```python
from build123d import *

# Parameters (mm, degrees)
SKETCH1_W           = 55
SKETCH1_H           = 13
BOSS_EXTRUDE1_DEPTH = 5
SKETCH2_R           = 4
BOSS_EXTRUDE2_DEPTH = 13
CUT_EXTRUDE1_REACH  = 63.016
SKETCH3_R           = 2.3


with BuildPart() as part:
    # Sketch1 → Boss-Extrude1 (new body)
    with BuildSketch(Plane(origin=(0, 0, 0), x_dir=(1, 0, 0), z_dir=(0, 1, 0))):
        with Locations((27.5, 6.5)):
            Rectangle(SKETCH1_W, SKETCH1_H)
    extrude(amount=BOSS_EXTRUDE1_DEPTH)

    # Sketch2 → Boss-Extrude2 (add)
    with BuildSketch(Plane.XY):
        with BuildLine():
            Line((13.5, 14), (13.5, 0))
            Line((13.5, 0), (41.5, 0))
            Line((41.5, 0), (41.5, 14))
            ThreePointArc((41.5, 14), (27.5, 28), (13.5, 14))
        make_face()
        with Locations((27.5, 14)):
            Circle(SKETCH2_R, mode=Mode.SUBTRACT)
    extrude(amount=-BOSS_EXTRUDE2_DEPTH)

    # Sketch3 → Cut-Extrude1 (cut, up to next)
    with BuildSketch(Plane(origin=(0, 5, 0), x_dir=(1, 0, 0), z_dir=(0, 1, 0)), mode=Mode.PRIVATE) as cut_extrude1_sk1:
        with Locations(Location((48.5, 6.5, 0), (0, 0, 270))):
            Circle(SKETCH3_R)
    cut_extrude1_tool1 = extrude(cut_extrude1_sk1.sketch, amount=-CUT_EXTRUDE1_REACH, mode=Mode.PRIVATE) & part.part
    # Sketch3 → Cut-Extrude1 (cut, up to next)
    with BuildSketch(Plane(origin=(0, 5, 0), x_dir=(1, 0, 0), z_dir=(0, 1, 0)), mode=Mode.PRIVATE) as cut_extrude1_sk2:
        with Locations(Location((6.5, 6.5, 0), (0, 0, 270))):
            Circle(SKETCH3_R)
    cut_extrude1_tool2 = extrude(cut_extrude1_sk2.sketch, amount=-CUT_EXTRUDE1_REACH, mode=Mode.PRIVATE) & part.part
    add(cut_extrude1_tool1.solids().sort_by_distance((48.5, 5, -6.5))[0], mode=Mode.SUBTRACT)
    add(cut_extrude1_tool2.solids().sort_by_distance((6.5, 5, -6.5))[0], mode=Mode.SUBTRACT)


solid = part.part
```
Read the model definition and answer for the solid it produces. Units are mm, in the model's axes. A direction names the side the tool comes from. Give positions to 0.01 mm unless a question says otherwise; leave off trailing zeros. Write each loop counter-clockwise with the first axis right and the second up, starting at its lowest first coordinate (ties: lowest second). Pieces come first, ordered by that corner, then holes. Notation, with made-up numbers: (72.25, 84) - (126.25, 84) arc R18 cw to (126.25, 91) - close; hole circle Ø8 at (21.5, 26). An arc over 180 degrees is marked (long way). Write item = value, one per line. Start each with the question number.
Item 1: Find section C-C (y = 11.25). Give the vertices of the cut face in (x, z).
Item 2: Each of these flat-tipped pins is pushed along its axis until it touches: P1, Ø4, axis at x = 46.5, z = -4.5, coming from the +Y side; P2, Ø2.5, axis at y = 9.5, z = -9, coming from the +X side; P3, Ø3.5, axis at x = 6.5, z = -6.5, coming from the -Y side; P4, Ø6, axis at y = 21.5, z = -9.5, coming from the -X side. Where does it stop, or does it pass through?
Item 3: Find section B-B (z = -6.5). Give the vertices of the cut face in (x, y), then the cut area to 3 significant figures.
Item 4: Find section A-A (x = 48.5). Give the vertices of the cut face in (y, z).
Item 5: The mould has two halves that part along X. Classify faces 3 (the flat face through (48, 5, -9)), 4 (the cylindrical face through (4.46, 2.54, -5.44)), 5 (the flat face through (41.5, 9, -6)), 6 (the flat face through (0, 2, -6)): +X half, -X half, draft (parallel to the pull), parting line (faces both ways), or undercut.
Item 6: Find the intervals of material crossed by probe 1 along X at (y, z) = (3.5, -6.5); probe 2 along Y at (x, z) = (27.5, -4); probe 3 along X at (y, z) = (5.25, -5.75), in increasing order. Write a range as [from, to].
Item 7: Find section D-D (z = -3.5). Give the vertices of the cut face in (x, y), then the cut area to 3 significant figures.
Item 8: A tool of negligible diameter and unlimited length cuts with its end or side. For faces 1 (the flat face through (27, 8, 0)), 2 (the flat face through (7, 5, -9)), from which of +Z, -Z, +X, -X, +Y, -Y can it reach the whole face along a straight path? Write none if from no direction.
Response:
q1.outline = (13.5, -13) - (24.6, -13) - (24.6, 0) - (13.5, 0) - close; (30.4, -13) - (41.5, -13) - (41.5, 0) - (30.4, 0) - close
q2.P1 = 5
q2.P2 = 41.5
q2.P3 = through
q2.P4 = 14.24
q3.outline = (0, 0) - (4.2, 0) - (4.2, 5) - (0, 5) - close; (8.8, 0) - (46.2, 0) - (46.2, 5) - (41.5, 5) - (41.5, 14) arc R14 ccw to (13.5, 14) - (13.5, 5) - (8.8, 5) - close; (50.8, 0) - (55, 0) - (55, 5) - (50.8, 5) - close; hole circle Ø8 at (27.5, 14)
q3.area = 739 mm²
q4.outline = (0, -13) - (5, -13) - (5, -8.8) - (0, -8.8) - close; (0, -4.2) - (5, -4.2) - (5, 0) - (0, 0) - close
q5.face_3 = draft
q5.face_4 = undercut
q5.face_5 = +X half
q5.face_6 = -X half
q6.probe_1 = [0, 4.2], [8.8, 46.2], [50.8, 55]
q6.probe_2 = [0, 10], [18, 28]
q6.probe_3 = [13.5, 41.5]
q7.outline = (0, 0) - (55, 0) - (55, 5) - (41.5, 5) - (41.5, 14) arc R14 ccw to (13.5, 14) - (13.5, 5) - (0, 5) - close; hole circle Ø8 at (27.5, 14)
q7.area = 785 mm²
q8.face_1 = +Z, +X, -X, +Y, -Y
q8.face_2 = +Z, -Z, -X, +Y
